Source: CAD feature listing. Evaluate the final solid. Frame: model axes, mm. A direction names the side the tool comes from. Give positions to 0.01 mm unless a question says otherwise; leave off trailing zeros. Order: outer loops, then holes, each group sorted by start corner. A loop starts at its lowest first (then second) coordinate and runs counter-clockwise, first axis right, second up. Notation, with made-up numbers: M -22,-20.75 L 32,-20.75 A35 ccw 32,14.25 Z; hole C -34.5,-5 d1. An arc over 180 degrees is marked long. Return JSON: item names as keys, results as strings.
from build123d import *

# Parameters (mm, degrees)
SKETCH1_W           = 120
SKETCH1_H           = 120
BOSS_EXTRUDE1_DEPTH = 6
SKETCH3_W           = 47.19594468
SKETCH3_H           = 11.33645236
BOSS_EXTRUDE2_DEPTH = 17.1
SKETCH4_W           = 16
SKETCH4_H           = 7
CUT_EXTRUDE3_DEPTH  = 106.01743865
SKETCH6_R           = 1.15
CUT_EXTRUDE4_DEPTH  = 8
FILLET1_R           = 4


with BuildPart() as part:
    # Sketch1 → Boss-Extrude1 (new body)
    with BuildSketch(Plane(origin=(0, 0, 0), x_dir=(0, 1, 0), z_dir=(0, 0, 1))):
        Rectangle(SKETCH1_W, SKETCH1_H)
    extrude(amount=BOSS_EXTRUDE1_DEPTH)

    # Sketch7 → CBORE for M3 SBHCS1 (revolve, cut)
    with BuildSketch(Plane(origin=(-55, 55, 6), x_dir=(0, -1, 0), z_dir=(1, 0, 0))):
        Polygon((0, 0), (0, 6), (1.25, 6), (1.25, 3), (3.25, 3), (3.25, 0.125), (3.375, 0), align=None)
    cbore_for_m3_sbhcs1 = revolve(axis=Axis((-55, 55, 12.35), (0, 0, -1)), mode=Mode.SUBTRACT)

    # Mirror2: CBORE for M3 SBHCS1 across plane
    add(cbore_for_m3_sbhcs1.mirror(Plane(origin=(0, 0, 0), x_dir=(0, 0, 1), z_dir=(1, 0, 0))), mode=Mode.SUBTRACT)

    # Mirror2 at the second plane: CBORE for M3 SBHCS1 across plane
    add(cbore_for_m3_sbhcs1.mirror(Plane.ZX), mode=Mode.SUBTRACT)

    # Mirror2 at the second plane copy 1 sketc → Mirror2 at the second plane copy 1 (revolve, cut)
    with BuildSketch(Plane(origin=(55, -55, 6), x_dir=(0, 1, 0), z_dir=(-1, 0, 0))):
        Polygon((0, 0), (0, 6), (1.25, 6), (1.25, 3), (3.25, 3), (3.25, 0.125), (3.375, 0), align=None)
    revolve(axis=Axis((55, -55, 12.35), (0, 0, -1)), mode=Mode.SUBTRACT)

    # Sketch3 → Boss-Extrude2 (add)
    with BuildSketch(Plane.XY.offset(6)):
        with Locations((0, -17.36822618)):
            Rectangle(SKETCH3_W, SKETCH3_H)
        with Locations((0, 17.36822618)):
            Rectangle(SKETCH3_W, SKETCH3_H)
    extrude(amount=BOSS_EXTRUDE2_DEPTH)

    # Sketch4 → Cut-Extrude3 (cut, through all)
    with BuildSketch(Plane.XZ.offset(23.03645236)):
        with Locations((0, 9.5)):
            Rectangle(SKETCH4_W, SKETCH4_H)
    extrude(amount=-CUT_EXTRUDE3_DEPTH, mode=Mode.SUBTRACT)

    # Sketch6 → Cut-Extrude4 (cut)
    with BuildSketch(Plane.XY.offset(23.1)):
        with Locations((0, 14.1)):
            Circle(SKETCH6_R)
        with Locations(Location((0, -14.1, 0), (0, 0, 180))):
            Circle(SKETCH6_R)
    extrude(amount=-CUT_EXTRUDE4_DEPTH, mode=Mode.SUBTRACT)

    # Fillet1
    fillet1_edges = [part.edges().sort_by_distance(p)[0] for p in [
        (-23.59797234, -17.36822618, 6),
        (23.59797234, -17.36822618, 6),
        (-23.59797234, -17.36822618, 23.1),
        (23.59797234, -17.36822618, 23.1),
        (-23.59797234, 17.36822618, 6),
        (23.59797234, 17.36822618, 6),
        (-23.59797234, 17.36822618, 23.1),
        (23.59797234, 17.36822618, 23.1),
    ]]
    fillet(fillet1_edges, radius=FILLET1_R)


solid = part.part
1. Ray query, probe 1 along X at (y, z) = (-55, 2.2); probe 2 along Y at (x, z) = (-55, 3.95). Return the intervals inside material, ascending.
Evaluation:
{"probe 1": "x = -60 to -56.25, -53.75 to 53.75, 56.25 to 60", "probe 2": "y = -60 to -58.25, -51.75 to 51.75, 58.25 to 60"}
2. Set-up query: faces 1 (the face through (-23.598, 17, 14)), 2 (the face through (8, 17, 9)), 3 (the face through (-53.022, 57.579, 4.458)). Return all of +Z, -Z, +X, -X, +Y, -Y with unobstructed straight access to the full face (end or side cutting, diameter ignored); none if empty.
Evaluation:
{"face 1": "+Z, -X, +Y, -Y", "face 2": "+Y, -Y", "face 3": "+Z"}
3. Draft query along Z for faces 4 (the face through (23.598, 17, 14)), 5 (the face through (0, 17, 23.1)), 6 (the face through (0, 17, 13)). Return one class per face: pulls with the +Z half, pulls with the -Z half, needs draft (parallel to the pull), parting line crosses it, or undercut.
Evaluation:
{"face 4": "needs draft", "face 5": "pulls with the +Z half", "face 6": "undercut"}
4. First-contact query: pin 1 (1.5 mm diameter, centred on x = -9.5, z = 15.5, fed in from +Y); pin 2 (1.2 mm diameter, centred on x = 0.5, y = 13.5, fed in from +Z); pin 3 (10 mm diameter, centred on y = -20, z = 15.5, fed in from +X); pin 4 (2 mm diameter, centred on x = -56, y = -56, fed in from +Z). Flat tips, straight axial feed; report the tip coordinate or a pass-through.
Evaluation:
{"pin 1": "stops at y = 23.04", "pin 2": "stops at z = 23.1", "pin 3": "stops at x = 23.6", "pin 4": "stops at z = 3"}
5. Section query D-D (x = 47.5). Return loops of the section in (y, z), then the cut area to 3 significant figures.
Evaluation:
{"outline": "M -60,0 L 60,0 L 60,6 L -60,6 Z", "area": "720 mm^2"}
6. Section query B-B (x = -6). Return loops of the section in (y, z).
Evaluation:
{"outline": "M -60,0 L 60,0 L 60,6 L -60,6 Z; M -23.04,13 L -11.7,13 L -11.7,23.1 L -23.04,23.1 Z; M 11.7,13 L 23.04,13 L 23.04,23.1 L 11.7,23.1 Z"}
7. Section query C-C (z = 8.5). Return loops of the section in (x, y), then the cut area to 3 significant figures.
Evaluation:
{"outline": "M -23.89,-23.04 L -8,-23.04 L -8,-11.7 L -23.89,-11.7 Z; M -23.89,11.7 L -8,11.7 L -8,23.04 L -23.89,23.04 Z; M 8,-23.04 L 23.89,-23.04 L 23.89,-11.7 L 8,-11.7 Z; M 8,11.7 L 23.89,11.7 L 23.89,23.04 L 8,23.04 Z", "area": "721 mm^2"}
8. Section query A-A (z = 17). Return loops of the section in (x, y), then the cut area to 3 significant figures.
Evaluation:
{"outline": "M -23.6,-23.04 L 23.6,-23.04 L 23.6,-11.7 L -23.6,-11.7 Z; M -23.6,11.7 L 23.6,11.7 L 23.6,23.04 L -23.6,23.04 Z; hole C 0,-14.1 d2.3; hole C 0,14.1 d2.3", "area": "1,060 mm^2"}
